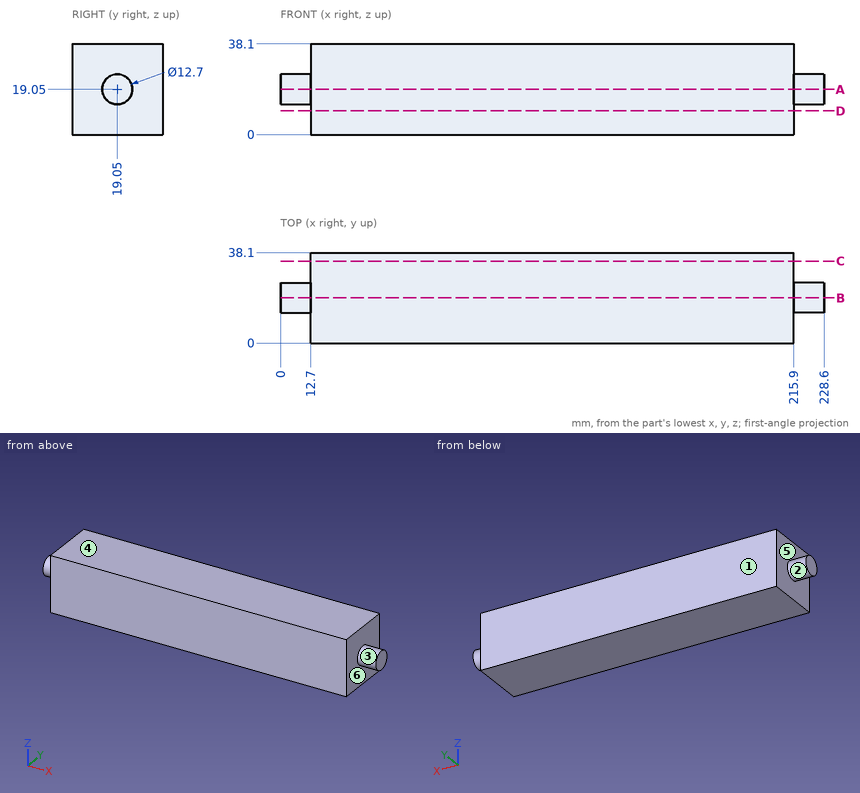
Input: dimensioned drawing with shaded views. Units: mm. Origin: part minimum x, y, z. A direction names the side the tool comes from. Give positions to 0.01 mm unless a question says otherwise; leave off trailing zeros. Order: outer loops, then holes, each group sorted by start corner. A loop starts at its lowest first (then second) coordinate and runs counter-clockwise, first axis right, second up. Notation, with made-up numbers: (-12.5, -4) -> (12.5, -4) arc R15 cw to (12.5, 5) -> close; hole circle Ø11 at (86, 25.25). An arc over 180 degrees is marked (long way). Use a Markdown table: item, result.
1) Contact query for flat-ended pins moving along their axis: P1, Ø10, axis at y = 9, z = 25, coming from the -X side; P2, Ø2, axis at x = 179, z = 6.5, coming from the -Y side; P3, Ø5, axis at y = 19.5, z = 5.5, coming from the +X side. Output: stop coordinate, or through.
Answer list:
| item | result |
|---|---|
| P1 | x = 12.7 |
| P2 | y = 0 |
| P3 | x = 215.9 |
2) Ray query, line 1 along X through (y, z) = (10, 32). Return the intervals inside material, ascending. Write a range as [from, to].
Answer list:
| item | result |
|---|---|
| line 1 | [12.7, 215.9] |
3) Section query A-A, the plane z = 19.05. Return the cut outline in (x, y), then the cut area to 3 significant figures.
Answer list:
| item | result |
|---|---|
| outline | (0, 12.7) -> (12.7, 12.7) -> (12.7, 0) -> (215.9, 0) -> (215.9, 12.7) -> (228.6, 12.7) -> (228.6, 25.4) -> (215.9, 25.4) -> (215.9, 38.1) -> (12.7, 38.1) -> (12.7, 25.4) -> (0, 25.4) -> close |
| area | 8,060 mm² |
4) Section query C-C, the plane y = 34.5. Return the cut outline in (x, z).
Answer list:
| item | result |
|---|---|
| outline | (12.7, 0) -> (215.9, 0) -> (215.9, 38.1) -> (12.7, 38.1) -> close |
5) Reachability of the marked faces 1, 2 and 3 from +Z, -Z, +X, -X, +Y, -Y: full face, straight path, thin tool, end or side. Return the list, or none.
Answer list:
| item | result |
|---|---|
| face 1 | +Z, -Z, +X, -X, +Y |
| face 2 | -X |
| face 3 | +X |
6) Mould query, pull axis X, two halves, no side actions, for the marked faces 4, 5 and 6. Classes: +X half, -X half, draft (parallel to the pull), parting line (faces both ways), or undercut.
Answer list:
| item | result |
|---|---|
| face 4 | draft |
| face 5 | -X half |
| face 6 | +X half |
